Verification items for the finished model (mm, model axes). A direction names the side the tool comes from. Round coordinates to 2 decimals unless told otherwise and drop trailing zeros. Order: outer loops, then holes, each group sorted by start corner. A loop starts at its lowest first (then second) coordinate and runs counter-clockwise, first axis right, second up. Notation, with made-up numbers: (11.5, 5.5) -> (45.5, 5.5) arc R21 cw to (45.5, 18.5) -> close; hole circle Ø9 at (20.5, 84.5). An arc over 180 degrees is marked (long way). Return JSON: item names as keys, results as strings. Group by question number.
1) Section check A-A on x = 16.5. Enter the section's corners in (y, z) (3 decimals).
2) Section check B-B on z = 214.5. Enter the section's corners in (x, y) (3 decimals).
3) Depth check by flat-ended pin: pin 1 (10 mm diameter, centred on y = 33, z = 320.5, fed in from +X) (3 decimals). Enter the tip coordinate at first touch or a pass-through.
4) Tool access check on faces 1 (the flat face through (3, 19, 0)), 2 (the flat face through (12, 3.175, 195)). Record the directions out of +Z, -Z, +X, -X, +Y, -Y that give a thin tool (end or side, any length) a straight path to the whole face; none if there is none.
5) Draft check along Y on faces 3 (the flat face through (3, 19, 395)), 4 (the flat face through (11, 41.326, 195)), 5 (the flat face through (3.175, 21, 195)). Enter one of: pulls with the +Y half, pulls with the -Y half, needs draft (parallel to the pull), parting line crosses it, or undercut.
6) Scan lines: L1, parallel to Y at x = 8.5, z = 254 (3 decimals); L2, parallel to X at y = 21, z = 219.5 (3 decimals). Record each from-to range of solid material in increasing order.
7) Section check C-C on y = 21.5. Enter the section's corners in (x, z) (3 decimals), plus the area to 3 significant figures.
Autodesk Fusion 360 part; units mm, degrees
sketch "Sketch1" plane through (0, 0, 0) normal (0, 0, 1) x (1, 0, 0)
  line L0 (0, 0) -> (21.0566, 0)
  line L1 (21.0566, 0) -> (21.0566, 41.3258)
  line L2 (21.0566, 41.3258) -> (0, 41.3258)
  line L3 (0, 41.3258) -> (0, 0)
  line L4 (0, 20.6629) -> (21.0566, 20.6629) construction
  line L5 (0, 38.1508) -> (21.0566, 38.1508)
  line L6 (21.0566, 38.1508) -> (21.0566, 3.175) construction
  line L7 (21.0566, 3.175) -> (0, 3.175)
  line L8 (0, 3.175) -> (0, 38.1508) construction
  line L9 (0, 38.1508) -> (21.0566, 3.175) construction
  line L10 (21.0566, 38.1508) -> (0, 3.175) construction
  line L11 (3.175, 38.1508) -> (3.175, 3.175)
  point P0 (10.5283, 20.6629)
  point P1 (0, 20.6629)
  dimension "d1" = 41.3258
  dimension "d2" = 21.0566
  dimension "d3" = 3.175
  dimension "d4" = 3.175
extrude "Extrude1" add sketch "Sketch1" along normal blind 395 contours L0 L1 L3 L7 | L3 L5 L7 L11 | L1 L2 L3 L5
sketch "Sketch2" plane through (0, 0, 395) normal (0, 0, 1) x (-1, 0, 0)
  line L0 (-21.0566, -38.1508) -> (-21.0566, -41.3258)
  line L1 (-21.0566, -41.3258) -> (0, -41.3258)
  line L2 (0, -41.3258) -> (0, 0)
  line L3 (0, 0) -> (-21.0566, 0)
  line L4 (-21.0566, 0) -> (-21.0566, -3.175)
  line L5 (-21.0566, -3.175) -> (-3.175, -3.175)
  line L6 (-3.175, -3.175) -> (-3.175, -38.1508)
  line L7 (-3.175, -38.1508) -> (-21.0566, -38.1508)
  point P0 (0, -20.6629)
Check result:
{
 "1": {"outline": "(0, 0) -> (3.175, 0) -> (3.175, 395) -> (0, 395) -> close; (38.151, 0) -> (41.326, 0) -> (41.326, 395) -> (38.151, 395) -> close"},
 "2": {"outline": "(0, 0) -> (21.057, 0) -> (21.057, 3.175) -> (3.175, 3.175) -> (3.175, 38.151) -> (21.057, 38.151) -> (21.057, 41.326) -> (0, 41.326) -> close"},
 "3": {"pin 1": "x = 3.175"},
 "4": {"face 1": "-Z, +X, -X, +Y, -Y", "face 2": "+Z, -Z, +X"},
 "5": {"face 3": "needs draft", "face 4": "pulls with the +Y half", "face 5": "undercut"},
 "6": {"L1": "0 to 3.175, 38.151 to 41.326", "L2": "0 to 3.175"},
 "7": {"outline": "(0, 0) -> (3.175, 0) -> (3.175, 395) -> (0, 395) -> close", "area": "1,250 mm^2"}
}
